```python
from build123d import *

# Parameters (mm, degrees)
SKETCH1_W           = 101.6
SKETCH1_H           = 50.8
BOSS_EXTRUDE1_DEPTH = 2.032
CUT_EXTRUDE1_DEPTH  = 3.032
LPATTERN1_COUNT     = 2
LPATTERN1_PITCH     = 25.4
LPATTERN1_COL_COUNT = 2
LPATTERN1_COL_PITCH = 25.4
SKETCH4_W           = 2.54
SKETCH4_H           = 50.8
BOSS_EXTRUDE2_DEPTH = 0.254


with BuildPart() as part:
    # Sketch1 → Boss-Extrude1 (new body)
    with BuildSketch(Plane(origin=(0, 0, 0), x_dir=(1, 0, 0), z_dir=(0, 1, 0))):
        Rectangle(SKETCH1_W, SKETCH1_H)
    extrude(amount=BOSS_EXTRUDE1_DEPTH)

    # Sketch2 → Cut-Extrude1 (cut, through all)
    with BuildSketch(Plane(origin=(0, 2.032, 0), x_dir=(1, 0, 0), z_dir=(0, 1, 0))):
        Polygon((-5.061841618, 7.282181714), (-2.790094674, 8.418300469), (-1.085916542, 5.010680054), (-3.357663485, 3.874561299), align=None)
    cut_extrude1 = extrude(amount=-CUT_EXTRUDE1_DEPTH, mode=Mode.SUBTRACT)

    # LPattern1: Cut-Extrude1 ×2
    with Locations(*[(-i * LPATTERN1_PITCH, 0, 0) for i in range(1, LPATTERN1_COUNT)]):
        add(cut_extrude1, mode=Mode.SUBTRACT)

    # LPattern1 col: Cut-Extrude1 ×2
    with Locations(*[(i * LPATTERN1_COL_PITCH, 0, 0) for i in range(1, LPATTERN1_COL_COUNT)]):
        add(cut_extrude1, mode=Mode.SUBTRACT)

    # Sketch4 → Boss-Extrude2 (add)
    with BuildSketch(Plane(origin=(0, 2.032, 0), x_dir=(1, 0, 0), z_dir=(0, 1, 0))):
        with Locations((-49.53, 0)):
            Rectangle(SKETCH4_W, SKETCH4_H)
        with Locations((49.53, 0)):
            Rectangle(SKETCH4_W, SKETCH4_H)
    extrude(amount=BOSS_EXTRUDE2_DEPTH)


solid = part.part
```
Verification items for the finished model (mm, model axes). A direction names the side the tool comes from. Give positions to 0.01 mm unless a question says otherwise; leave off trailing zeros. Order: outer loops, then holes, each group sorted by start corner. A loop starts at its lowest first (then second) coordinate and runs counter-clockwise, first axis right, second up. Notation, with made-up numbers: M 73.25,40 L 128.25,40 A13 cw 128.25,54 Z; hole C -22.5,-26.5 d7. An arc over 180 degrees is marked long. Return JSON: item names as keys, results as strings. Group by question number.
1) Mould release check, pull along Z, two halves, no side actions. Record for faces 1 (the face through (23.19, 1.03, -4.45)), 2 (the face through (-50.8, 1, 0)), 3 (the face through (23.45, 1.03, -6.74)), 4 (the face through (-1, 1, -25.4)): pulls with the +Z half, pulls with the -Z half, needs draft (parallel to the pull), parting line crosses it, or undercut.
2) Go/stop test with a flat-tipped pin: pin 1 Ø3 at (x, z) = (8.5, 6.5) entering from +Y. Record where the tip stops, or that it passes through.
3) Section check B-B on x = -25.5. Record the cut outline in (y, z).
4) Scan lines: line 1 (X direction, y = 2.1, z = 21.5); line 2 (Y direction, x = -33.5, z = -23); line 3 (Z direction, x = 22.5, y = 0.7). Record each from-to range of solid material in increasing order.
5) Section check A-A on z = -10.5. Record the cut outline in (x, y), and give its area (3 significant figures).
6) Access from +Z, -Z, +X, -X, +Y, -Y to the whole of each face (thin tool, end or side, straight path). Record for faces 5 (the face through (-29.342, 1.03, -7.842)), 6 (the face through (-1, 1, 25.4)).
Answer block:
{
 "1": {"face 1": "undercut", "face 2": "needs draft", "face 3": "undercut", "face 4": "pulls with the -Z half"},
 "2": {"pin 1": "stops at y = 2.03"},
 "3": {"outline": "M 0,-25.4 L 2.03,-25.4 L 2.03,25.4 L 0,25.4 Z"},
 "4": {"line 1": "x = -50.8 to -48.26, 48.26 to 50.8", "line 2": "y = 0 to 2.03", "line 3": "z = -25.4 to -8.36, -4.1 to 25.4"},
 "5": {"outline": "M -50.8,0 L 50.8,0 L 50.8,2.29 L 48.26,2.29 L 48.26,2.03 L -48.26,2.03 L -48.26,2.29 L -50.8,2.29 Z", "area": "208 mm^2"},
 "6": {"face 5": "+Y, -Y", "face 6": "+Z, +X, -X, +Y, -Y"}
}
